Geometry: final body of the model. Coordinates: model frame, mm. Give positions to 0.01 mm unless a question says otherwise; leave off trailing zeros. Write each loop counter-clockwise with the first axis right and the second up, starting at its lowest first coordinate (ties: lowest second). Pieces come first, ordered by that corner, then holes. Notation, with made-up numbers: M -26,62.5 L 22,62.5 A8 cw 22,72.5 Z; hole C 49,-31 d2. An arc over 180 degrees is marked long. Use one line per item in the form item = value. Start each with the question number.
Item 1: Material intervals for line 1 along Y through (x, z) = (80, 0.6); line 2 along X through (y, z) = (-10, 0.85); line 3 along X through (y, z) = (-9.5, 1.1), sorted ascending. Write a range as from..to.
Item 2: Pull-direction query (X, two-part tool) for faces 1 (the cylindrical face through (26.75, -10.08, 0.81)), 2 (the flat face through (44, -30, 0)), 3 (the cylindrical face through (7.129, -52.482, 0.811)); classes: released by +X, released by -X, zero draft, split by the parting line, or undercut.
Item 3: Section query B-B on y = -54.5. Return loops of the section in (x, z).
Item 4: Section query A-A on z = 0.7. Return loops of the section in (x, y), then the cut area to 3 significant figures.
Autodesk Fusion 360 part; units mm, degrees
sketch "Sketch4" plane through (0, 0, 0) normal (0, 0, 1) x (1, 0, 0)
  line L0 (0, 0) -> (90, 0)
  line L1 (90, 0) -> (90, -60)
  line L2 (90, -60) -> (0, -60)
  line L3 (0, -60) -> (0, 0)
  dimension "d13" = 90
  dimension "d14" = 60
extrude "Extrude3" add sketch "Sketch4" along normal blind 1.6
fillet "Fillet1" radius 25 2 edges at (0, -60, 0.8) (0, 0, 0.8)
fillet "Fillet2" radius 10 2 edges at (90, -60, 0.8) (90, 0, 0.8)
sketch "Sketch5" plane through (0, 0, 1.6) normal (0, 0, 1) x (-1, 0, 0)
  arc A0 (-90, 10) -> (-80, 0) centre (-80, 10) ccw
  line L0 (-80, 0) -> (-25, 0)
  arc A1 (-25, 0) -> (0, 25) centre (-25, 25) ccw
  line L1 (0, 25) -> (0, 35)
  arc A2 (0, 35) -> (-25, 60) centre (-25, 35) ccw
  line L2 (-25, 60) -> (-80, 60)
  arc A3 (-80, 60) -> (-90, 50) centre (-80, 50) ccw
  line L3 (-90, 50) -> (-90, 10)
  line L4 (-80, 10) -> (-25, 10)
  line L5 (-25, 10) -> (-25, 50)
  line L6 (-25, 50) -> (-80, 50)
  line L7 (-80, 50) -> (-80, 10)
  circle A4 centre (-80, 10) radius 1.75
  circle A5 centre (-25, 10) radius 1.75
  circle A6 centre (-25, 50) radius 1.75
  circle A7 centre (-80, 50) radius 1.75
  dimension "d21" = 3.5
  dimension "d22" = 3.5
  dimension "d23" = 3.5
  dimension "d24" = 3.5
extrude "Extrude4" cut sketch "Sketch5" against normal blind 2 contours L4 L7 A4 | L4 L7 A4 | L4 L5 A5 | L4 L5 A5 | L6 L7 A7 | L6 L7 A7 | L5 L6 A6 | L5 L6 A6
sketch "Sketch6" plane through (0, 0, 1.6) normal (0, 0, 1) x (-1, 0, 0)
  circle A0 centre (-80, 10) radius 1.75
  circle A1 centre (-80, 50) radius 1.75
  circle A2 centre (-25, 10) radius 1.75
  circle A3 centre (-25, 50) radius 1.75
  arc A4 (-90, 10) -> (-80, 0) centre (-80, 10) ccw
  line L0 (-80, 0) -> (-25, 0)
  arc A5 (-25, 0) -> (0, 25) centre (-25, 25) ccw
  line L1 (0, 25) -> (0, 35)
  arc A6 (0, 35) -> (-25, 60) centre (-25, 35) ccw
  line L2 (-25, 60) -> (-80, 60)
  arc A7 (-80, 60) -> (-90, 50) centre (-80, 50) ccw
  line L3 (-90, 50) -> (-90, 10)
sketch "Sketch7" plane through (0, 0, 1.6) normal (0, 0, 1) x (-1, 0, 0)
  circle A0 centre (-80, 10) radius 1.75
  circle A1 centre (-80, 50) radius 1.75
  circle A2 centre (-25, 10) radius 1.75
  circle A3 centre (-25, 50) radius 1.75
  arc A4 (-90, 10) -> (-80, 0) centre (-80, 10) ccw
  line L0 (-80, 0) -> (-25, 0)
  arc A5 (-25, 0) -> (0, 25) centre (-25, 25) ccw
  line L1 (0, 25) -> (0, 35)
  arc A6 (0, 35) -> (-25, 60) centre (-25, 35) ccw
  line L2 (-25, 60) -> (-80, 60)
  arc A7 (-80, 60) -> (-90, 50) centre (-80, 50) ccw
  line L3 (-90, 50) -> (-90, 10)
Answer sheet:
q1.line_1 = -60..-51.75, -48.25..-11.75, -8.25..0
q1.line_2 = 5..23.25, 26.75..78.25, 81.75..90
q1.line_3 = 5.38..23.32, 26.68..78.32, 81.68..89.99
q2.face_1 = undercut
q2.face_2 = zero draft
q2.face_3 = released by -X
q3.outline = M 9.36,0 L 88.93,0 L 88.93,1.6 L 9.36,1.6 Z
q4.outline = M 0,-35 A25 ccw 25,-60 L 80,-60 A10 ccw 90,-50 L 90,-10 A10 ccw 80,0 L 25,0 A25 ccw 0,-25 Z; hole C 25,-50 d3.5; hole C 25,-10 d3.5; hole C 80,-50 d3.5; hole C 80,-10 d3.5
q4.area = 5,050 mm2
